```python
from build123d import *

# Parameters (mm, degrees)
F0_W     = 5
F0_H     = 10
F1_DEPTH = 5


# Not quite as in the source:
# - a feature names something its author has since deleted; it is built from what else it names


with BuildPart() as f1:
    # F0 (on Right) → F1 (new body)
    with BuildSketch(Plane.YZ):
        Polygon((0, 59.5256769704), (0, 0), (250, 0), (250, 200), (151.1586640426, 360.9612668205), (-117.4855289776, 355.6046891351), (-145.3168663312, 248.8862540722), (129.4880870227, 248.8862540722), (129.4880870227, 239.8862540722), (-111.9774808093, 239.8862540722), (-111.9774808093, 207.8862540722), (-41.9774808093, 207.8862540722), (-41.9774808093, 198.8862540722), (-111.9774808093, 198.8862540722), (-113.683141768, 136.7378532887), align=None)
        with Locations((3.0250263214, 158.6281073093)):
            Rectangle(F0_W, F0_H, mode=Mode.SUBTRACT)
        with Locations((28.0250263214, 158.6281073093)):
            Rectangle(F0_W, F0_H, mode=Mode.SUBTRACT)
        with Locations((63.0250263214, 158.6281073093)):
            Rectangle(F0_W, F0_H, mode=Mode.SUBTRACT)
        with Locations((88.0250263214, 158.6281073093)):
            Rectangle(F0_W, F0_H, mode=Mode.SUBTRACT)
        with Locations((3.0250263214, 193.6281073093)):
            Rectangle(F0_W, F0_H, mode=Mode.SUBTRACT)
        with Locations((28.0250263214, 193.6281073093)):
            Rectangle(F0_W, F0_H, mode=Mode.SUBTRACT)
        with Locations((-99.690104425, 278.8862540722)):
            Rectangle(F0_W, F0_H, mode=Mode.SUBTRACT)
        with Locations((-99.690104425, 313.8862540722)):
            Rectangle(F0_W, F0_H, mode=Mode.SUBTRACT)
        with Locations((-74.690104425, 278.8862540722)):
            Rectangle(F0_W, F0_H, mode=Mode.SUBTRACT)
        with Locations((-74.690104425, 313.8862540722)):
            Rectangle(F0_W, F0_H, mode=Mode.SUBTRACT)
        with Locations((-39.690104425, 278.8862540722)):
            Rectangle(F0_W, F0_H, mode=Mode.SUBTRACT)
        with Locations((-14.690104425, 278.8862540722)):
            Rectangle(F0_W, F0_H, mode=Mode.SUBTRACT)
        with Locations((-39.690104425, 313.8862540722)):
            Rectangle(F0_W, F0_H, mode=Mode.SUBTRACT)
        with Locations((-14.690104425, 313.8862540722)):
            Rectangle(F0_W, F0_H, mode=Mode.SUBTRACT)
        with Locations((63.0250263214, 193.6281073093)):
            Rectangle(F0_W, F0_H, mode=Mode.SUBTRACT)
        with Locations((88.0250263214, 193.6281073093)):
            Rectangle(F0_W, F0_H, mode=Mode.SUBTRACT)
    extrude(amount=F1_DEPTH)


solid = f1.part
```
Work out the finished part from the listing and answer in its coordinate system (mm). Coordinates: 2 decimals unless noted, no trailing zeros. Loops run counter-clockwise (first coordinate to the right, second up) from the corner with the lowest first, then second, coordinate; pieces in that order, holes last. Notation, with made-up numbers: M -22,88 L -18,88 A12 ccw -18,102 Z; hole C -30.75,74.25 d5. An arc over 180 degrees is marked long. Use CSV: the item, a comma, the result in double quotes. Start each with the question number.
(1) Find section D-D, the plane y = 215. Give the vertices of the cut face in (x, z), then the cut area to 3 significant figures.
(2) Consider line 1 (Z direction, x = 1.55, y = -14.5); line 2 (Z direction, x = 4.5, y = -111); line 3 (Z direction, x = 2.4, y = -39.5). Determine where each line is inside the solid, lowest interval first.
(3) Find section B-B, the plane x = 2.85. State how many separate pieces and enclosed holes the cut face has, then the cut area to 3 significant figures.
(4) Find section A-A, the plane z = 193.5. Give the vertices of the cut face in (x, y).
(5) Find section C-C, the plane z = 28. Give the vertices of the cut face in (x, y).
(6) Given pin 1 Ø1.5 at (x, y) = (3, -15) entering from -Z; pin 2 Ø2.5 at (x, z) = (3, 281.5) entering from +Y; pin 3 Ø2 at (x, z) = (1, 279) entering from +Y, each flat-ended and moving along its own axis, determine where each tip first touches the part or whether it passes through.
Recorded:
1,outline,"M 0,0 L 5,0 L 5,257 L 0,257 Z"
1,area,"1,280 mm^2"
2,line 1,"z = 69.37 to 239.89, 248.89 to 273.89, 283.89 to 308.89, 318.89 to 357.66"
2,line 2,"z = 134.92 to 198.89, 207.89 to 239.89, 248.89 to 355.73"
2,line 3,"z = 86.35 to 239.89, 248.89 to 273.89, 283.89 to 308.89, 318.89 to 357.16"
3,separate pieces,"1"
3,enclosed holes,"16"
3,area,"110,000 mm^2"
4,outline,"M 0,-112.13 L 5,-112.13 L 5,0.53 L 0,0.53 Z; M 0,5.53 L 5,5.53 L 5,25.53 L 0,25.53 Z; M 0,30.53 L 5,30.53 L 5,60.53 L 0,60.53 Z; M 0,65.53 L 5,65.53 L 5,85.53 L 0,85.53 Z; M 0,90.53 L 5,90.53 L 5,250 L 0,250 Z"
5,outline,"M 0,0 L 5,0 L 5,250 L 0,250 Z"
6,pin 1,"stops at z = 69.2"
6,pin 2,"stops at y = 200.72"
6,pin 3,"stops at y = 202.1"
